Here's how the part is built. I have some questions about the finished solid (model axes, mm). A direction names the side the tool comes from. Coordinates: 2 decimals unless noted, no trailing zeros. Write each loop counter-clockwise with the first axis right and the second up, starting at its lowest first coordinate (ties: lowest second). Pieces come first, ordered by that corner, then holes.
Item 1: For faces 1 (the face through (4.54, 98.51, -131.44)), 2 (the face through (4.44, -98.51, -131.54)), 3 (the face through (6.35, -98, -77)), which set-ups out of +Z, -Z, +X, -X, +Y, -Y let a thin tool reach every point of the face, with its end or its side?
Item 2: I'm going to push flat-ended pins straight in: P1, Ø1, axis at x = -4, z = -133.5, coming from the +Y side (3 decimals); P2, Ø10, axis at y = 98, z = -55, coming from the -X side. Where does each tip first touch, or does it pass through?
Item 3: I want a section at A-A (z = -96). Please give me the cut outline in (x, y) (3 decimals), and give its area (3 significant figures).
Item 4: Please list where these lines run through material, in increasing order: line 1 (Y direction, x = -8, z = -99) (3 decimals); line 2 (Z direction, x = -2.25, y = -92.5).
from build123d import *

# Parameters (mm, degrees)
F0_W     = 19.05
F0_H     = 184.15
F1_DEPTH = 152.4
F2_W     = 12.7
F2_H     = 114.3
F3_DEPTH = 12.7
F4_W     = 12.7
F4_H     = 114.3
F5_DEPTH = 12.7
F6_R     = 6.34999


# Not quite as in the source:
# - a fillet or chamfer is up to 0.001 mm smaller than in the source, because OpenCascade refuses the exact size


with BuildPart() as f1:
    # F0 (on Top) → F1 (new body)
    with BuildSketch(Plane.XY):
        Rectangle(F0_W, F0_H)
    extrude(amount=-F1_DEPTH)

    # F2 (on face) → F3 (join)
    with BuildSketch(Plane.XZ.offset(92.075)):
        with Locations((0, -76.2)):
            Rectangle(F2_W, F2_H)
    extrude(amount=F3_DEPTH)

    # F4 (on face) → F5 (join)
    with BuildSketch(Plane(origin=(0, 92.075, 0), x_dir=(-1, 0, 0), z_dir=(0, 1, 0))):
        with Locations((0, -76.2)):
            Rectangle(F4_W, F4_H)
    extrude(amount=F5_DEPTH)

    # F6 (radius 6.35 in the source; OpenCascade refuses exactly that, so slightly less here)
    f6_edges = [f1.edges().sort_by_distance(p)[0] for p in [
        (6.35, 98.425, -19.05),
        (-6.35, 98.425, -19.05),
        (-6.35, 98.425, -133.35),
        (6.35, 98.425, -133.35),
        (-6.35, -98.425, -19.05),
        (6.35, -98.425, -19.05),
        (-6.35, -98.425, -133.35),
        (6.35, -98.425, -133.35),
    ]]
    fillet(f6_edges, radius=F6_R)


solid = f1.part
Answer:
1. face 1: -Z, +X, +Y
1. face 2: -Z, +X, -Y
1. face 3: +Z, -Z, +X, -Y
2. P1: stops at y = 92.075
2. P2: stops at x = -6.35
3. outline: (-9.525, -92.075) - (-6.35, -92.075) - (-6.35, -104.775) - (6.35, -104.775) - (6.35, -92.075) - (9.525, -92.075) - (9.525, 92.075) - (6.35, 92.075) - (6.35, 104.775) - (-6.35, 104.775) - (-6.35, 92.075) - (-9.525, 92.075) - close
3. area: 3,830 mm2
4. line 1: y = -92.075 to 92.075
4. line 2: z = -132.94 to -19.46
